Verification items for this drawing (mm, ordinates from the low corner). A direction names the side the tool comes from. Round coordinates to 2 decimals unless told otherwise and drop trailing zeros. Loops run counter-clockwise (first coordinate to the right, second up) from the corner with the lowest first, then second, coordinate; pieces in that order, holes last. Notation, with made-up numbers: M -24.5,3.25 L -3.5,3.25 A4 ccw -3.5,7.25 Z; hole C -2.5,86.5 d8. An arc over 180 degrees is marked long. Write item = value, one per line. Start each with the question number.
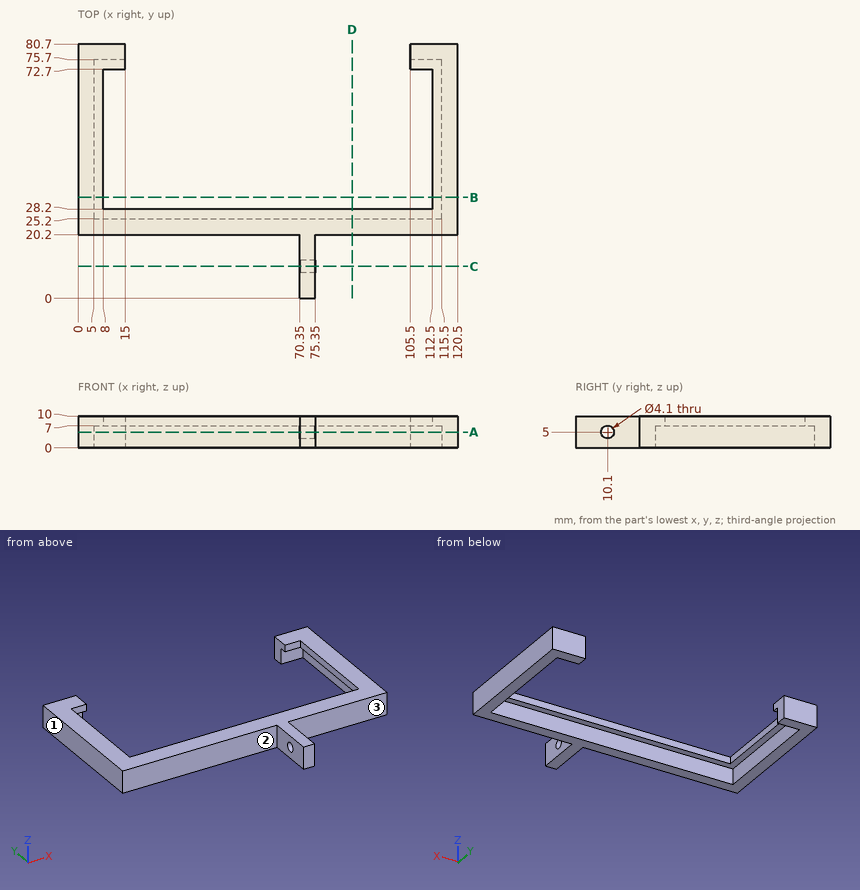
1. Gauge pin test, flat ends, axial feed: P1, Ø1.5, axis at x = 89, z = 8, coming from the -Y side; P2, Ø5, axis at y = 8.5, z = 4.5, coming from the +X side; P3, Ø2, axis at x = 73.5, z = 4, coming from the +Y side; P4, Ø3.5, axis at y = 10.1, z = 5, coming from the +X side. Record the tip position at first contact, or that the pin passes through.
2. Section check D-D, the plane x = 87. Enter the section's corners in (y, z).
3. Tool access check on the marked faces 1, 2 and 3. Record the directions out of +Z, -Z, +X, -X, +Y, -Y that give a thin tool (end or side, any length) a straight path to the whole face; none if there is none.
4. Section check A-A, the plane z = 5. Enter the section's corners in (x, y).
5. Section check B-B, the plane y = 32. Enter the section's corners in (x, z).
6. Section check C-C, the plane y = 10.1. Enter the section's corners in (x, z), and give its area (3 significant figures).
7. Thickness scan on line 1 (Z direction, x = 73, y = 10); line 2 (Y direction, x = 109, z = 6.25); line 3 (X direction, y = 37, z = 5.5). Record the ranges inside material, lowest first.
Computed values:
q1.P1 = 20.2
q1.P2 = 75.35
q1.P3 = 25.2
q1.P4 = through
q2.outline = M 20.2,0 L 25.2,0 L 25.2,7 L 28.2,7 L 28.2,10 L 20.2,10 Z
q3.face_1 = +Z, -Z, -X, +Y, -Y
q3.face_2 = +Z, -Z, -X, -Y
q3.face_3 = +Z, -Z, +X, -Y
q4.outline = M 0,20.2 L 70.35,20.2 L 70.35,12.15 L 75.35,12.15 L 75.35,20.2 L 120.5,20.2 L 120.5,80.7 L 105.5,80.7 L 105.5,75.7 L 115.5,75.7 L 115.5,25.2 L 5,25.2 L 5,75.7 L 15,75.7 L 15,80.7 L 0,80.7 Z; M 70.35,0 L 75.35,0 L 75.35,8.05 L 70.35,8.05 Z
q5.outline = M 0,0 L 5,0 L 5,7 L 8,7 L 8,10 L 0,10 Z; M 112.5,7 L 115.5,7 L 115.5,0 L 120.5,0 L 120.5,10 L 112.5,10 Z
q6.outline = M 70.35,0 L 75.35,0 L 75.35,2.95 L 70.35,2.95 Z; M 70.35,7.05 L 75.35,7.05 L 75.35,10 L 70.35,10 Z
q6.area = 29.5 mm2
q7.line_1 = 0 to 2.95, 7.05 to 10
q7.line_2 = 20.2 to 25.2, 75.7 to 80.7
q7.line_3 = 0 to 5, 115.5 to 120.5
